Input: part model. Units: mm. Frame: model coordinates. Face numbers are marked on the shaded views. A direction names the side the tool comes from. Coordinates: 2 decimals unless noted, no trailing zeros. Loops run counter-clockwise (first coordinate to the right, second up) from the corner with the lowest first, then second, coordinate; pieces in that order, holes last.
(1) Section B-B, the plane z = 3. Return loops of the section in (x, y).
(2) Mould query, pull axis Z, two halves, no side actions, for the marked faces 1, 2, 3 and 4. Classes: released by +Z, released by -Z, zero draft, split by the parting line, or undercut.
(3) Set-up query: the marked faces 5, 6 and 7. Return all of +Z, -Z, +X, -X, +Y, -Y with unobstructed straight access to the full face (end or side cutting, diameter ignored); none if empty.
(4) Contact query for flat-ended pins moving along their axis: P1, Ø3.5, axis at x = -0.5, z = 10, coming from the -Y side; P2, Ø9.5, axis at x = -2.5, z = 42.5, coming from the +Y side; P3, Ø8, axis at x = -4, y = -11, coming from the -Z side. Output: stop coordinate, or through.
(5) Section A-A, the plane z = 45.2. Return loops of the section in (x, y), then the cut area to 3 significant figures.
(6) Line query: L1, parallel to X at y = 1.75, z = 45.2; L2, parallel to Z at x = -4.5, y = -4.5; L3, parallel to X at y = -4, z = 45. Output: solid intervals per line, ascending.
(7) Section C-C, the plane y = 3.25. Return loops of the section in (x, z), then the cut area to 3 significant figures.
(8) Section D-D, the plane x = 0. Return loops of the section in (y, z).
Autodesk Inventor part; units mm, degrees
ref_plane "YZ Plane" through (0, 0, 0) normal (1, 0, 0) x (0, 1, 0)
ref_plane "XZ Plane" through (0, 0, 0) normal (0, 1, 0) x (-1, 0, 0)
ref_plane "XY Plane" through (0, 0, 0) normal (0, 0, 1) x (1, 0, 0)
sketch "草图1" plane through (0, 0, 0) normal (0, 0, 1) x (1, 0, 0)
  line L0 (-5, 0) -> (5, 0) construction
  line L1 (-5, -6.3307) -> (5, -6.3307)
  line L2 (5, 5.4693) -> (-5, 5.4693)
  arc A0 (-5, 5.4693) -> (-5, -6.3307) centre (-1.0059, -0.4307) ccw
  line L3 (0, 0) -> (0, 3.0217)
  arc A1 (5, -6.3307) -> (5, 5.4693) centre (1.0059, -0.4307) ccw
  line L4 (5, 5.4693) -> (5, -6.3307)
  line L5 (-5, 5.4693) -> (-5, -6.3307)
  point P0 (-10.9, 0)
  point P1 (10.9, 0)
  point P2 (10.9, 0)
  dimension "d0" = 11.8
  dimension "d6" = 10
extrude "拉伸1" add sketch "草图1" along normal blind 29
sketch "草图2" plane through (0, 0, 29) normal (0, 0, 1) x (1, 0, 0)
  line L0 (6, -5.4307) -> (-6, -5.4307)
  line L1 (-6, -5.4307) -> (-6, 4.5693)
  line L2 (-6, 4.5693) -> (6, 4.5693)
  line L3 (6, 4.5693) -> (6, -5.4307)
  line L4 (6, -5.4307) -> (-6, 4.5693) construction
  line L5 (-6, -5.4307) -> (6, 4.5693) construction
  line L6 (5, 5.4693) -> (-5, 5.4693)
  line L7 (0, 5.4693) -> (0, -6.3307)
  line L8 (-5, -6.3307) -> (5, -6.3307)
  point P0 (0, -0.4307)
  dimension "d4" = 10
  dimension "d5" = 12
extrude "拉伸2" add sketch "草图2" along normal blind 18
sketch "草图3" plane through (0, 0, 0) normal (0, 0, -1) x (-1, 0, 0)
  line L0 (5, -6.3307) -> (-5, -6.3307)
  arc A0 (5, -6.3307) -> (5, 5.4693) centre (1.0059, -0.4307) ccw
  line L1 (-5, 5.4693) -> (5, 5.4693)
  arc A1 (-5, 5.4693) -> (-5, -6.3307) centre (-1.0059, -0.4307) ccw
  arc A2 (5.2957, -7.3307) -> (5.2957, 6.4693) centre (1.0059, -0.4307) ccw
  line L2 (5.2957, -7.3307) -> (-5.2957, -7.3307)
  arc A3 (-5.2957, 6.4693) -> (-5.2957, -7.3307) centre (-1.0059, -0.4307) ccw
  line L3 (-5.2957, 6.4693) -> (5.2957, 6.4693)
  line L4 (-9.1307, -0.4307) -> (9.1307, -0.4307)
  line L5 (9.1307, -0.4307) -> (9.1307, -12.0307)
  line L6 (9.1307, -12.0307) -> (-9.1307, -12.0307)
  line L7 (-9.1307, -12.0307) -> (-9.1307, -0.4307)
  point P0 (0, 0)
  dimension "d9" = 1
  dimension "d10" = 18.5
extrude "拉伸3" add sketch "草图3" along normal blind 1
sketch "草图4" plane through (0, 0, -1) normal (0, 0, -1) x (-1, 0, 0)
  circle A0 centre (0, 0) radius 5.5587
extrude "拉伸4" add sketch "草图4" along normal blind 2
sketch "草图5" plane through (-6, -5.4307, 29) normal (0, 1, 0) x (1, 0, 0)
  circle A0 centre (6, -14) radius 1.5
  line L0 (12, -18) -> (0, -18)
  point P0 (6, 29)
  dimension "d15" = 4
  dimension "d16" = 3
extrude "拉伸5" add sketch "草图5" against normal blind 8
sketch "草图7" plane through (0, -13.4307, 43) normal (0, -1, 0) x (1, 0, 0)
  circle A0 centre (0, 0) radius 1.5
  line L0 (-1.118, 1) -> (1.118, 1)
  point P0 (0, -43)
  point P1 (0, 1.5)
  dimension "d19" = 0.5
extrude "拉伸6" cut sketch "草图7" against normal up to surface (8 mm away) contours L0 A0 picked at (-0.0599, 1.1631)
fillet "圆角1" radius 4 4 edges at (-5, 5.4693, 14.5) (5, 5.4693, 14.5) (-5, -6.3307, 14.5) (5, -6.3307, 14.5)
fillet "圆角2" radius 3 2 edges at (-9.1307, -12.0307, -0.5) (9.1307, -12.0307, -0.5)
sketch "草图8" plane through (-6, -5.4307, 29) normal (0, -1, 0) x (1, 0, 0)
  circle A0 centre (10.0294, 16.2) radius 0.7
  circle A1 centre (1.5294, 16.2) radius 0.7
  line L0 (0, 18) -> (12, 18)
  point P0 (6, -29)
  dimension "d24" = 1.4
  dimension "d25" = 1.4
  dimension "d26" = 8.5
  dimension "d27" = 1.8
extrude "拉伸7" cut sketch "草图8" against normal blind 11.75
properties part number "电机"
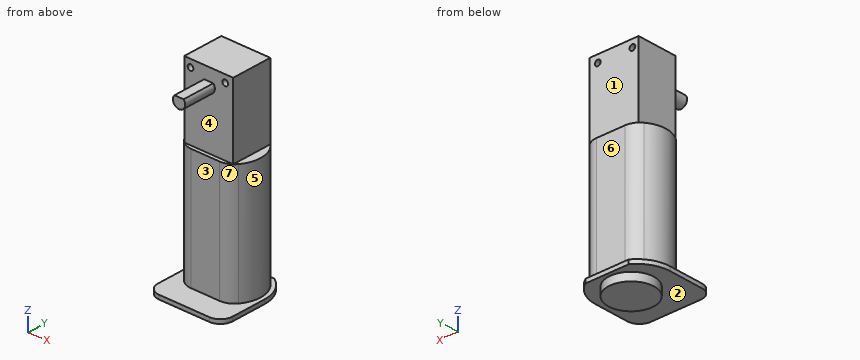
Report:
1. outline: (-6.66, -4.76) arc R4 ccw to (-3.49, -6.33) - (3.49, -6.33) arc R4 ccw to (6.66, -4.76) arc R7.12 ccw to (6.66, 3.9) arc R4 ccw to (3.49, 5.47) - (-3.49, 5.47) arc R4 ccw to (-6.66, 3.9) arc R7.12 ccw to start
2. face 1: zero draft
2. face 2: released by -Z
2. face 3: undercut
2. face 4: undercut
3. face 5: +Z, +X
3. face 6: +Z, +X, -X, +Y
3. face 7: +Z, +X, -Y
4. P1: stops at y = -6.33
4. P2: stops at y = 4.57
4. P3: stops at z = -1
5. outline: (-6, -5.43) - (-5.17, -5.43) - (-5.17, 4.57) - (-6, 4.57) - close; (-3.77, -5.43) - (3.33, -5.43) - (3.33, 4.57) - (-3.77, 4.57) - close; (4.73, -5.43) - (6, -5.43) - (6, 4.57) - (4.73, 4.57) - close
5. area: 92.0 mm2
6. L1: x = -6 to -5.17, -3.77 to 3.33, 4.73 to 6
6. L2: z = -1 to 44.5, 45.9 to 47
6. L3: x = -6 to -5.14, -3.8 to 3.36, 4.7 to 6
7. outline: (-8.25, -1) - (-4.51, -1) - (-4.51, -3) - (4.51, -3) - (4.51, -1) - (8.25, -1) - (8.25, 0) - (7.11, 0) - (7.11, 29) - (6, 29) - (6, 47) - (-6, 47) - (-6, 29) - (-7.11, 29) - (-7.11, 0) - (-8.25, 0) - close; hole circle Ø1.4 at (-4.47, 45.2); hole circle Ø1.4 at (4.03, 45.2)
7. area: 660 mm2
8. outline: (-13.43, 41.5) - (-5.43, 41.5) - (-5.43, 29) - (-6.33, 29) - (-6.33, 0) - (-12.03, 0) - (-12.03, -1) - (-5.56, -1) - (-5.56, -3) - (5.56, -3) - (5.56, -1) - (6.47, -1) - (6.47, 0) - (5.47, 0) - (5.47, 29) - (4.57, 29) - (4.57, 47) - (-5.43, 47) - (-5.43, 44) - (-13.43, 44) - close
